For this review, use the dimensioned drawing (mm, ordinates from the lowest corner) and the shaded views. Give positions to 0.01 mm unless a question says otherwise; leave off trailing zeros. Loops run counter-clockwise (first coordinate to the right, second up) from the corner with the lowest first, then second, coordinate; pieces in that order, holes last. Notation, with made-up numbers: M 34.25,-5 L 63.25,-5 A18 ccw 63.25,13 Z; hole C 9,32.25 d9. An arc over 180 degrees is marked long. Use CSV: the item, a comma, the result in double quotes. Start each with the question number.
1. Take a section at A-A, the plane y = 173. Write out the cut boundary in (x, z), and give its area (3 significant figures).
2. Insertion check: P1, Ø3, axis at x = 501.5, z = 294, coming from the +Y side; P2, Ø20.5, axis at x = 355.5, y = 340.5, coming from the -Z side; P3, Ø7.5, axis at x = 174.5, z = 309, coming from the -Y side. Each pin has a flat end and moves straight along its axis. Give the tip position at first contact, or say it passes through.
3. Take a section at C-C, the plane x = 289. Write out the cut boundary in (y, z), and give its area (3 significant figures).
4. Take a section at B-B, the plane z = 98. Write out the cut boundary in (x, y), and give its area (3 significant figures).
5. To check wall thickness, follow line 1 (X direction, y = 184, z = 161); line 2 (Z direction, x = 390, y = 328.5). State the ranges of each line that lie inside material, in increasing order. Write a range as [from, to].
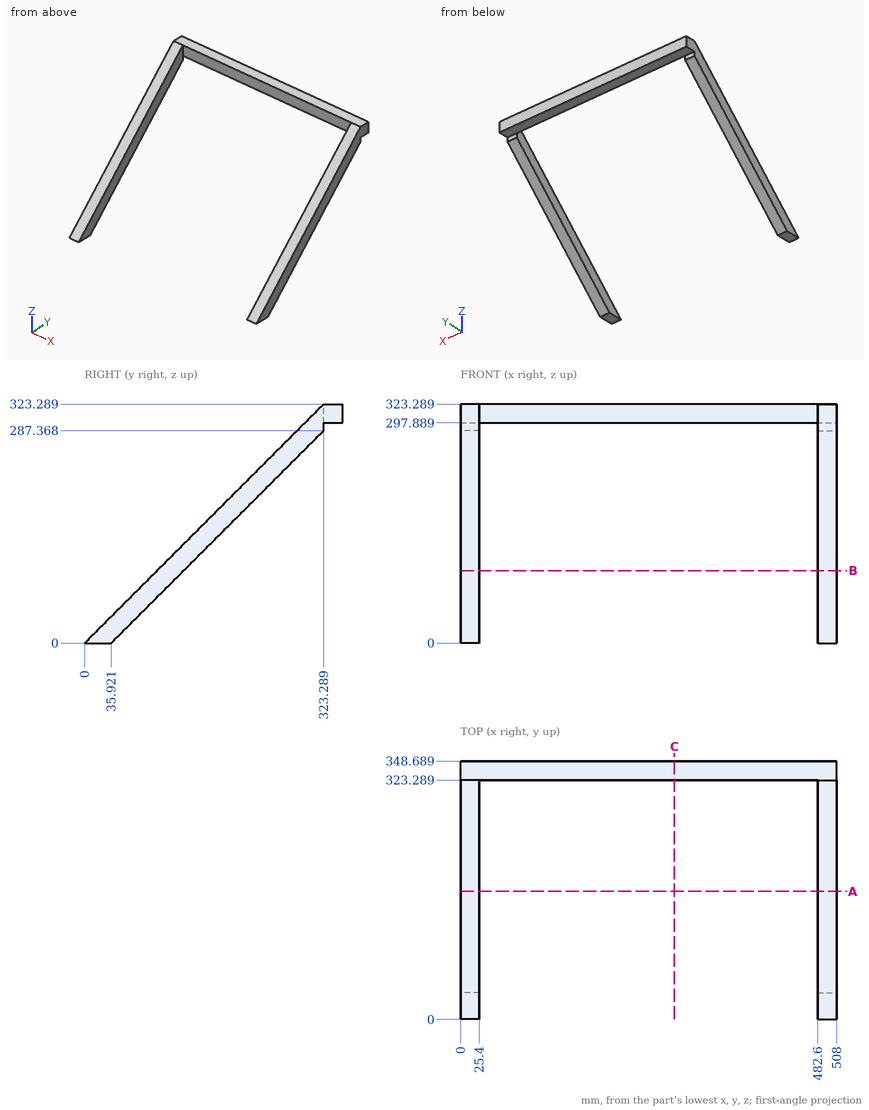
Result set:
1,outline,"M 0,137.08 L 25.4,137.08 L 25.4,173 L 0,173 Z; M 482.6,137.08 L 508,137.08 L 508,173 L 482.6,173 Z"
1,area,"1,820 mm2"
2,P1,"y = 323.29"
2,P2,"z = 297.89"
2,P3,"y = 323.29"
3,outline,"M 323.29,297.89 L 348.69,297.89 L 348.69,323.29 L 323.29,323.29 Z"
3,area,"645 mm2"
4,outline,"M 0,98 L 25.4,98 L 25.4,133.92 L 0,133.92 Z; M 482.6,98 L 508,98 L 508,133.92 L 482.6,133.92 Z"
4,area,"1,820 mm2"
5,line 1,"[0, 25.4], [482.6, 508]"
5,line 2,"[297.89, 323.29]"
